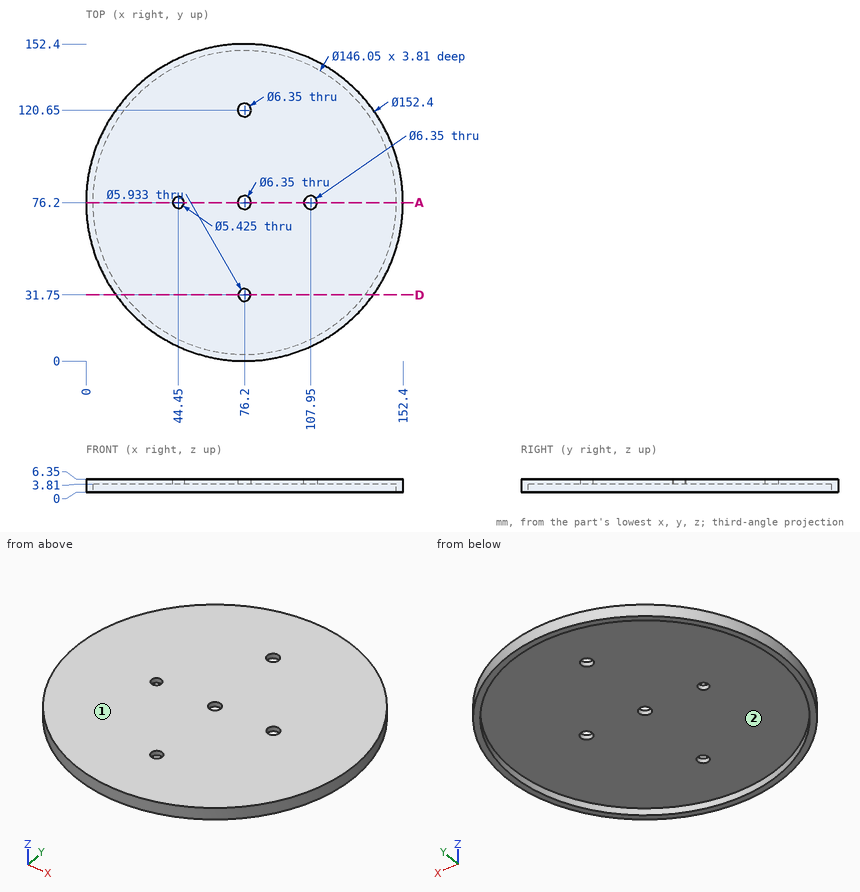
Print and shaded views of the part. All mm, measured from the part's lowest x, y and z. Coordinates: 2 decimals unless noted, no trailing zeros. Write each loop counter-clockwise with the first axis right and the second up, starting at its lowest first coordinate (ties: lowest second). Pieces come first, ordered by that corner, then holes. Notation, with made-up numbers: M 79.5,14 L 110.5,14 A29 ccw 110.5,42 Z; hole C 29.5,22.25 d2. An arc over 180 degrees is marked long. Return JSON: item names as keys, results as strings.
1. Saw through at A-A, the plane y = 76.2. Count the separate pieces of the cut face and the enclosed holes in it, then the cut area to 3 significant figures.
Determined:
{"separate pieces": "4", "enclosed holes": "0", "area": "365 mm²"}
2. Flat gauge pins, fed straight in: pin 1 Ø2 at (x, z) = (88.5, 5) entering from +Y; pin 2 Ø2 at (y, z) = (37.5, 1.5) entering from +X; pin 3 Ø5.5 at (x, y) = (76.2, 31.75) entering from -Z; pin 4 Ø7.5 at (x, y) = (107.95, 76.2) entering from +Z. Where does each tip first touch, or does it go through?
Determined:
{"pin 1": "y = 151.56", "pin 2": "x = 142.42", "pin 3": "through", "pin 4": "z = 6.35"}
3. Probe L1, parallel to Y at x = 76.2, z = 4.5 (1 decimal); L2, parallel to Y at x = 77, z = 5 (1 decimal); L3, parallel to Z at x = 142.5, y = 54. List the from-to ranges inside material, lowest first.
Determined:
{"L1": "0 to 28.8, 34.7 to 73, 79.4 to 117.5, 123.8 to 152.4", "L2": "0 to 28.9, 34.6 to 73.1, 79.3 to 117.6, 123.7 to 152.4", "L3": "3.81 to 6.35"}
4. Pull direction X, two halves, no side cores. Call the marked faces 1 and 2: pulls with the +X half, pulls with the -X half, needs draft (parallel to the pull), parting line crosses it, or undercut.
Determined:
{"face 1": "needs draft", "face 2": "undercut"}
5. Saw through at D-D, the plane y = 31.75. Write the cut outline in (x, z).
Determined:
{"outline": "M 14.31,0 L 18.26,0 L 18.26,3.81 L 73.23,3.81 L 73.23,6.35 L 14.31,6.35 Z; M 79.17,3.81 L 134.14,3.81 L 134.14,0 L 138.09,0 L 138.09,6.35 L 79.17,6.35 Z"}
